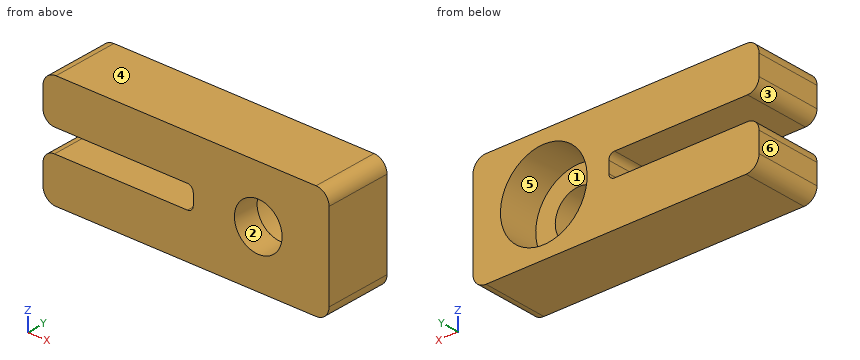
```python
from build123d import *

# Parameters (mm, degrees)
SKETCH_1_R          = 1.65
EXTRUDE_1_DEPTH     = 4.6
CUT_EXTRUDE_1_DEPTH = 4.6
FILLET_1_R          = 0.8
SKETCH_3_R          = 3
CUT_EXTRUDE_2_DEPTH = 2.8


with BuildPart() as part:
    # 草图1 → 凸台-拉伸1 (new body)
    with BuildSketch(Plane(origin=(0, 0, 0), x_dir=(1, 0, 0), z_dir=(0, 1, 0))):
        with BuildLine():
            Line((-9.9, -3), (-9.9, 3))
            ThreePointArc((-9.9, 3), (-9.636396103, 3.636396103), (-9, 3.9))
            Line((-9, 3.9), (9, 3.9))
            ThreePointArc((9, 3.9), (9.636396103, 3.636396103), (9.9, 3))
            Line((9.9, 3), (9.9, -3))
            ThreePointArc((9.9, -3), (9.636396103, -3.636396103), (9, -3.9))
            Line((9, -3.9), (-9, -3.9))
            ThreePointArc((-9, -3.9), (-9.636396103, -3.636396103), (-9.9, -3))
        make_face()
        with Locations(Location((5, 0, 0), (0, 0, 270))):
            Circle(SKETCH_1_R, mode=Mode.SUBTRACT)
    extrude(amount=EXTRUDE_1_DEPTH)

    # 草图2 → 切除-拉伸1 (cut)
    with BuildSketch(Plane(origin=(0, 4.6, 0), x_dir=(1, 0, 0), z_dir=(0, 1, 0))):
        with BuildLine():
            Line((-10.1, 0.8), (0.1, 0.8))
            ThreePointArc((0.1, 0.8), (0.382842712, 0.682842712), (0.5, 0.4))
            Line((0.5, 0.4), (0.5, -0.4))
            ThreePointArc((0.5, -0.4), (0.382842712, -0.682842712), (0.1, -0.8))
            Line((0.1, -0.8), (-10.1, -0.8))
            ThreePointArc((-10.1, -0.8), (-10.382842712, -0.682842712), (-10.5, -0.4))
            Line((-10.5, -0.4), (-10.5, 0.4))
            ThreePointArc((-10.5, 0.4), (-10.382842712, 0.682842712), (-10.1, 0.8))
        make_face()
    extrude(amount=-CUT_EXTRUDE_1_DEPTH, mode=Mode.SUBTRACT)

    # 圆角1
    fillet_1_edges = [part.edges().sort_by_distance(p)[0] for p in [
        (-9.9, 2.3, 0.8),
        (-9.9, 2.3, -0.8),
    ]]
    fillet(fillet_1_edges, radius=FILLET_1_R)

    # 草图3 → 切除-拉伸2 (cut)
    with BuildSketch(Plane(origin=(0, 4.6, 0), x_dir=(1, 0, 0), z_dir=(0, 1, 0))):
        with Locations(Location((5, 0, 0), (0, 0, 270))):
            Circle(SKETCH_3_R)
    extrude(amount=-CUT_EXTRUDE_2_DEPTH, mode=Mode.SUBTRACT)


solid = part.part
```
Geometry check sheet. Reference: the model listing, model coordinates, mm. Face numbers are marked on the shaded views. A direction names the side the tool comes from. Coordinates: 2 decimals unless noted, no trailing zeros. Order: outer loops, then holes, each group sorted by start corner. A loop starts at its lowest first (then second) coordinate and runs counter-clockwise, first axis right, second up.
Item 1: Section check B-B (z = 0). Enter the section's corners in (x, y).
Item 2: Mould release check, pull along Z, two halves, no side actions. Record for the marked faces 4, 5 and 6: released by +Z, released by -Z, zero draft, split by the parting line, or undercut.
Item 3: Section check A-A (y = 1). Enter the section's corners in (x, z).
Item 4: Section check C-C (x = -3.5). Enter the section's corners in (y, z), plus the area to 3 significant figures.
Item 5: Depth check by flat-ended pin: pin 1 (3 mm diameter, centred on x = 4.5, z = -0.5, fed in from +Y); pin 2 (4 mm diameter, centred on x = 2.5, z = -2, fed in from -Y). Enter the tip coordinate at first touch or a pass-through.
Item 6: Section check D-D (x = 5). Enter the section's corners in (y, z), plus the area to 3 significant figures.
Item 7: Tool access check on the marked faces 1, 2 and 3. Record the directions out of +Z, -Z, +X, -X, +Y, -Y that give a thin tool (end or side, any length) a straight path to the whole face; none if there is none.
Item 8: Scan lines: line 1 along X through (y, z) = (0.8, 0); line 2 along Z through (x, y) = (5, 0.5); line 3 along X through (y, z) = (3.3, 0). Record each from-to range of solid material in increasing order.
Check sheet entries:
1. outline: (0.5, 0) - (3.35, 0) - (3.35, 1.8) - (2, 1.8) - (2, 4.6) - (0.5, 4.6) - close; (6.65, 0) - (9.9, 0) - (9.9, 4.6) - (8, 4.6) - (8, 1.8) - (6.65, 1.8) - close
2. face 4: released by +Z
2. face 5: undercut
2. face 6: zero draft
3. outline: (-9.9, -3) arc R0.9 ccw to (-9, -3.9) - (9, -3.9) arc R0.9 ccw to (9.9, -3) - (9.9, 3) arc R0.9 ccw to (9, 3.9) - (-9, 3.9) arc R0.9 ccw to (-9.9, 3) - (-9.9, 1.6) arc R0.8 ccw to (-9.1, 0.8) - (0.1, 0.8) arc R0.4 cw to (0.5, 0.4) - (0.5, -0.4) arc R0.4 cw to (0.1, -0.8) - (-9.1, -0.8) arc R0.8 ccw to (-9.9, -1.6) - close; hole circle Ø3.3 at (5, 0)
4. outline: (0, -3.9) - (4.6, -3.9) - (4.6, -0.8) - (0, -0.8) - close; (0, 0.8) - (4.6, 0.8) - (4.6, 3.9) - (0, 3.9) - close
4. area: 28.5 mm2
5. pin 1: stops at y = 1.8
5. pin 2: stops at y = 0
6. outline: (0, -3.9) - (4.6, -3.9) - (4.6, -3) - (1.8, -3) - (1.8, -1.65) - (0, -1.65) - close; (0, 1.65) - (1.8, 1.65) - (1.8, 3) - (4.6, 3) - (4.6, 3.9) - (0, 3.9) - close
6. area: 13.1 mm2
7. face 1: +Y
7. face 2: +Y, -Y
7. face 3: -X, +Y, -Y
8. line 1: x = 0.5 to 3.35, 6.65 to 9.9
8. line 2: z = -3.9 to -1.65, 1.65 to 3.9
8. line 3: x = 0.5 to 2, 8 to 9.9
